Input: dimensioned drawing with shaded views. Units: mm. Origin: part minimum x, y, z. A direction names the side the tool comes from. Coordinates: 2 decimals unless noted, no trailing zeros. Loops run counter-clockwise (first coordinate to the right, second up) from the corner with the lowest first, then second, coordinate; pieces in that order, holes last.
Item 1: Pull-direction query (X, two-part tool) for the marked faces 1, 2 and 3; classes: +X half, -X half, draft (parallel to the pull), parting line (faces both ways), or undercut.
Item 2: Reachability of the marked faces 4, 5 and 6 from +Z, -Z, +X, -X, +Y, -Y: full face, straight path, thin tool, end or side. Return the list, or none.
Item 3: Section query C-C, the plane z = 15. Return the cut outline in (x, y).
Item 4: Section query B-B, the plane y = 46.3. Return the cut outline in (x, z), then the cut area to 3 significant figures.
Item 5: Section query D-D, the plane x = 16.5. Return the cut outline in (y, z).
Item 6: Line query: probe 1 along X at (y, z) = (46.3, 24); probe 2 along Z at (x, y) = (6.5, 26); probe 3 along X at (y, z) = (26, 11.5). Output: solid intervals per line, ascending.
Item 7: Section query A-A, the plane y = 12. Return the cut outline in (x, z), then the cut area to 3 significant figures.
Item 8: Pin query (flat end, axial travel): pin 1 Ø10 at (x, y) = (26, 7.5) entering from -Z; pin 2 Ø3.5 at (x, y) = (5, 33) entering from -Z; pin 3 Ø1 at (x, y) = (3.499, 30) entering from +Z; pin 4 Ø6 at (y, z) = (7, 15) entering from -X. Return the tip coordinate at first contact, or that it passes through.
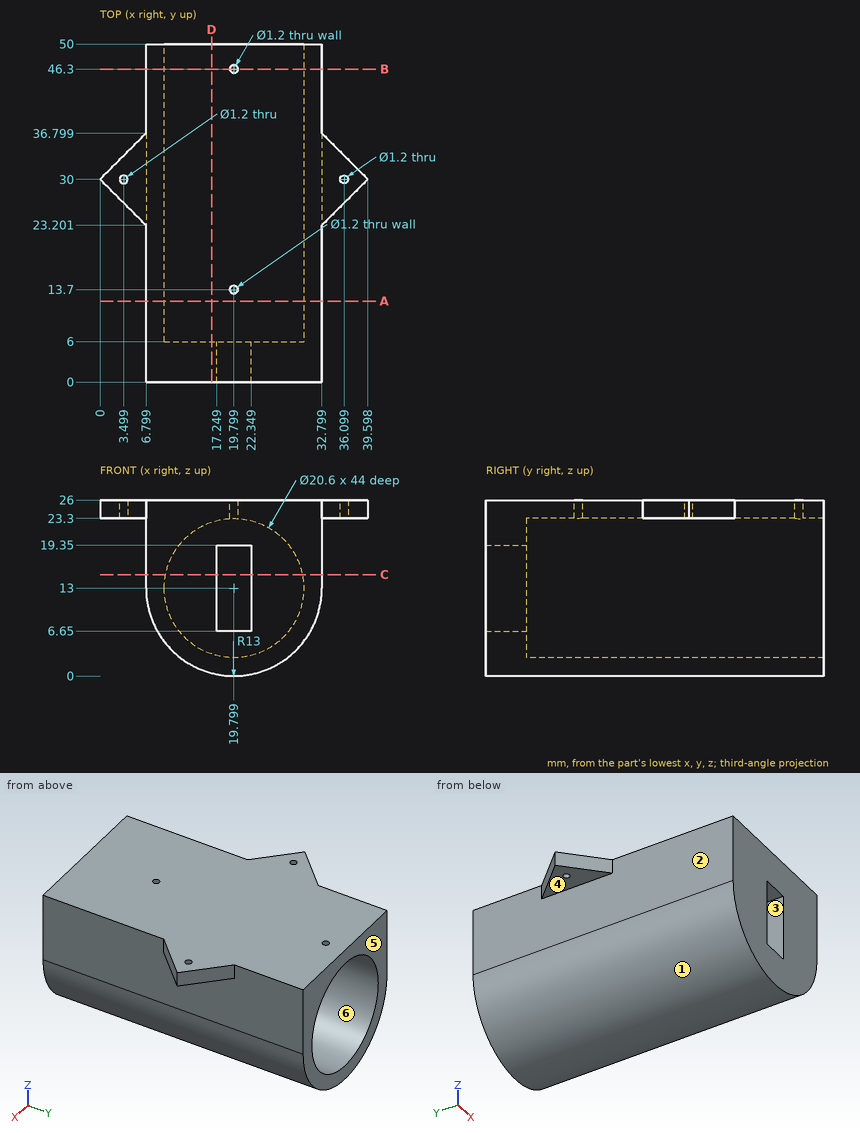
Verdict:
1. face 1: parting line
1. face 2: -X half
1. face 3: undercut
2. face 4: -Z, -X, +Y, -Y
2. face 5: +Z, -Z, +X, -X, +Y
2. face 6: +Y
3. outline: (6.8, 0) - (17.25, 0) - (17.25, 6) - (9.7, 6) - (9.7, 50) - (6.8, 50) - close; (22.35, 0) - (32.8, 0) - (32.8, 50) - (29.9, 50) - (29.9, 6) - (22.35, 6) - close
4. outline: (6.8, 13) arc R13 ccw to (32.8, 13) - (32.8, 26) - (20.4, 26) - (20.4, 23.28) arc R10.3 cw (long way) to (19.2, 23.28) - (19.2, 26) - (6.8, 26) - close
4. area: 267 mm2
5. outline: (0, 0.43) - (50, 0.43) - (50, 3.24) - (6, 3.24) - (6, 22.76) - (50, 22.76) - (50, 26) - (0, 26) - close
6. probe 1: x = 6.8 to 19.2, 20.4 to 32.8
6. probe 2: z = 23.3 to 26
6. probe 3: x = 6.89 to 9.61, 29.99 to 32.71
7. outline: (6.8, 13) arc R13 ccw to (32.8, 13) - (32.8, 26) - (6.8, 26) - close; hole circle Ø20.6 at (19.8, 13)
7. area: 270 mm2
8. pin 1: stops at z = 0.06
8. pin 2: stops at z = 23.3
8. pin 3: passes through
8. pin 4: stops at x = 6.8
